Drawing for the job (mm, zero at the part's lowest x, y, z). Round coordinates to 2 decimals unless told otherwise and drop trailing zeros. Loops run counter-clockwise (first coordinate to the right, second up) from the corner with the lowest first, then second, coordinate; pieces in that order, holes last. Notation, with made-up numbers: (-18, 61) -> (-12, 61) arc R20 ccw to (-12, 100) -> close; hole circle Ø1 at (-13, -37). An arc over 180 degrees is marked (long way). Put each result on its own line as item: value. Start each with the question number.
Item 1: Cut at D-D, the plane x = 68. List the corners of the cut face in (y, z) (1 decimal).
Item 2: Cut at B-B, the plane y = 10.16. List the corners of the cut face in (x, z) (1 decimal), plus the area to 3 significant figures.
Item 3: Cut at A-A, the plane y = 35.56. List the corners of the cut face in (x, z) (1 decimal).
Item 4: Cut at C-C, the plane z = 1.05. List the corners of the cut face in (x, y) (1 decimal), plus the area to 3 significant figures.
Item 5: Drill centre lines: probe 1 along Y at (x, z) = (43, 2.15); probe 2 along X at (y, z) = (9.5, 1.95) (1 decimal); probe 3 along X at (y, z) = (10.5, 1.05) (1 decimal). Where is each one in solid material? Low to high. Write a range as [from, to].
Item 6: Flat gauge pins, fed straight in: pin 1 Ø4 at (x, y) = (8.001, 35.56) entering from -Z; pin 2 Ø1 at (x, z) = (36, 1.5) entering from +Y. Where does each tip first touch, or does it go through?
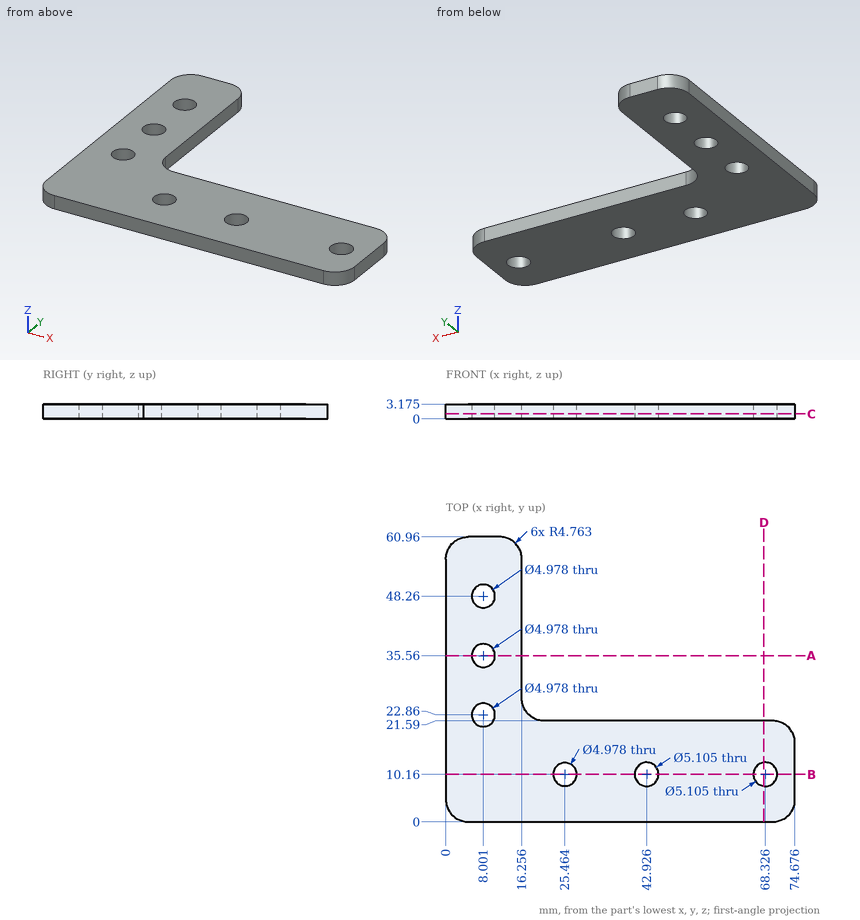
Reply:
1. outline: (0, 0) -> (7.6, 0) -> (7.6, 3.2) -> (0, 3.2) -> close; (12.7, 0) -> (21.6, 0) -> (21.6, 3.2) -> (12.7, 3.2) -> close
2. outline: (0, 0) -> (23, 0) -> (23, 3.2) -> (0, 3.2) -> close; (28, 0) -> (40.4, 0) -> (40.4, 3.2) -> (28, 3.2) -> close; (45.5, 0) -> (65.8, 0) -> (65.8, 3.2) -> (45.5, 3.2) -> close; (70.9, 0) -> (74.7, 0) -> (74.7, 3.2) -> (70.9, 3.2) -> close
2. area: 189 mm^2
3. outline: (0, 0) -> (5.5, 0) -> (5.5, 3.2) -> (0, 3.2) -> close; (10.5, 0) -> (16.3, 0) -> (16.3, 3.2) -> (10.5, 3.2) -> close
4. outline: (0, 4.8) arc R4.8 ccw to (4.8, 0) -> (69.9, 0) arc R4.8 ccw to (74.7, 4.8) -> (74.7, 16.8) arc R4.8 ccw to (69.9, 21.6) -> (21, 21.6) arc R4.8 cw to (16.3, 26.4) -> (16.3, 56.2) arc R4.8 ccw to (11.5, 61) -> (4.8, 61) arc R4.8 ccw to (0, 56.2) -> close; hole circle Ø5 at (8, 22.9); hole circle Ø5 at (8, 35.6); hole circle Ø5 at (8, 48.3); hole circle Ø5 at (25.5, 10.2); hole circle Ø5.1 at (42.9, 10.2); hole circle Ø5.1 at (68.3, 10.2)
4. area: 2,110 mm^2
5. probe 1: y = [0, 7.61], [12.71, 21.59]
5. probe 2: x = [0, 23.1], [27.9, 40.5], [45.4, 65.9], [70.8, 74.7]
5. probe 3: x = [0, 23], [27.9, 40.4], [45.5, 65.8], [70.9, 74.7]
6. pin 1: passes through
6. pin 2: stops at y = 21.59
